Part model, mm, in its own coordinate system. Round coordinates to 2 decimals unless told otherwise and drop trailing zeros. Loops run counter-clockwise (first coordinate to the right, second up) from the corner with the lowest first, then second, coordinate; pieces in that order, holes last.
from build123d import *

# Parameters (mm, degrees)
SKETCH1_R           = 14.5
BOSS_EXTRUDE1_DEPTH = 50
SKETCH2_R           = 1.1
CUT_EXTRUDE1_DEPTH  = 47
CHAMFER1_SIZE       = 0.5


with BuildPart() as part:
    # Sketch1 → Boss-Extrude1 (new body)
    with BuildSketch(Plane(origin=(0, 0, 0), x_dir=(1, 0, 0), z_dir=(0, 1, 0))):
        with Locations(Location((0, 0, 0), (0, 0, 270))):
            Circle(SKETCH1_R)
    extrude(amount=BOSS_EXTRUDE1_DEPTH)

    # Sketch2 → Cut-Extrude1 (cut)
    with BuildSketch(Plane.XZ):
        with BuildLine():
            Line((-12.75, 0.9), (-12.75, -0.9))
            Line((-12.75, -0.9), (-11.638182396, -0.9))
            ThreePointArc((-11.638182396, -0.9), (-12.005537317, -1.66663011), (-12.573189655, -2.299435125))
            ThreePointArc((-12.573189655, -2.299435125), (-9.280361808, -8.789049136), (-2.979270067, -12.429660087))
            ThreePointArc((-2.979270067, -12.429660087), (0, -9.781725236), (2.979270067, -12.429660087))
            ThreePointArc((2.979270067, -12.429660087), (9.280361808, -8.789049136), (12.573189655, -2.299435125))
            ThreePointArc((12.573189655, -2.299435125), (12.005537317, -1.66663011), (11.638182396, -0.9))
            Line((11.638182396, -0.9), (12.75, -0.9))
            Line((12.75, -0.9), (12.75, 0.9))
            Line((12.75, 0.9), (11.638182396, 0.9))
            ThreePointArc((11.638182396, 0.9), (12.005537317, 1.66663011), (12.573189655, 2.299435125))
            ThreePointArc((12.573189655, 2.299435125), (9.280361808, 8.789049136), (2.979270067, 12.429660087))
            ThreePointArc((2.979270067, 12.429660087), (0, 9.781725236), (-2.979270067, 12.429660087))
            ThreePointArc((-2.979270067, 12.429660087), (-9.280361808, 8.789049136), (-12.573189655, 2.299435125))
            ThreePointArc((-12.573189655, 2.299435125), (-12.005537317, 1.66663011), (-11.638182396, 0.9))
            Line((-11.638182396, 0.9), (-12.75, 0.9))
        make_face()
        with Locations(Location((0, -12.781725236, 0), (0, 0, 270))):
            Circle(SKETCH2_R)
        with Locations(Location((0, 12.781725236, 0), (0, 0, 270))):
            Circle(SKETCH2_R)
    extrude(amount=-CUT_EXTRUDE1_DEPTH, mode=Mode.SUBTRACT)

    # Chamfer1
    chamfer1_edges = [part.edges().sort_by_distance(p)[0] for p in [
        (9.280361808, 47, 8.789049136),
        (0, 0, -14.5),
        (12.75, 47, 0),
        (-9.280361808, 47, -8.789049136),
        (-12.75, 47, 0),
        (-9.280361808, 0, -8.789049136),
        (9.280361808, 0, -8.789049136),
        (9.280361808, 0, 8.789049136),
        (-9.280361808, 0, 8.789049136),
        (0, 50, -14.5),
    ]]
    chamfer(chamfer1_edges, length=CHAMFER1_SIZE)


solid = part.part
1) Drop flat-ended pins along their axis: pin 1 Ø5 at (y, z) = (30.5, -4) entering from +X; pin 2 Ø4 at (y, z) = (28, 8.5) entering from -X; pin 3 Ø3 at (x, z) = (-4.5, 3) entering from -Y. Give the stop position or say it passes through.
Values:
pin 1: stops at x = 14.42
pin 2: stops at x = -12.96
pin 3: stops at y = 47
2) Slice it at B-B, the plane z = 0. Give the cut face in (x, y).
Values:
outline: (-14.5, 0.5) - (-14, 0) - (-12.75, 0) - (-12.75, 46.5) - (-12.25, 47) - (12.25, 47) - (12.75, 46.5) - (12.75, 0) - (14, 0) - (14.5, 0.5) - (14.5, 49.5) - (14, 50) - (-14, 50) - (-14.5, 49.5) - close
3) Slice it at C-C, the plane x = 0. Give the cut face in (y, z), then the cut area to 3 significant figures.
Values:
outline: (0, -14) - (0.5, -14.5) - (49.5, -14.5) - (50, -14) - (50, 14) - (49.5, 14.5) - (0.5, 14.5) - (0, 14) - (0, 13.88) - (47, 13.88) - (47, 11.68) - (0, 11.68) - (0, 9.78) - (47, 9.78) - (47, -9.78) - (0, -9.78) - (0, -11.68) - (47, -11.68) - (47, -13.88) - (0, -13.88) - close
area: 323 mm2
4) Slice it at A-A, the plane y = 19. Give the cut face in (x, z).
Values:
outline: circle Ø29 at (0, 0); hole (-12.75, -0.9) - (-11.64, -0.9) arc R3 cw to (-12.57, -2.3) arc R12.78 ccw to (-2.98, -12.43) arc R3 cw to (2.98, -12.43) arc R12.78 ccw to (12.57, -2.3) arc R3 cw to (11.64, -0.9) - (12.75, -0.9) - (12.75, 0.9) - (11.64, 0.9) arc R3 cw to (12.57, 2.3) arc R12.78 ccw to (2.98, 12.43) arc R3 cw to (-2.98, 12.43) arc R12.78 ccw to (-12.57, 2.3) arc R3 cw to (-11.64, 0.9) - (-12.75, 0.9) - close; hole circle Ø2.2 at (0, -12.78); hole circle Ø2.2 at (0, 12.78)
5) Wall check: line 1 along X through (y, z) = (35.5, 2.5); line 2 along X through (y, z) = (37.5, 4.75); line 3 along Z through (x, y) = (4, 18). Give the ranges that are in metal, low to high.
Values:
line 1: x = -14.28 to -12.53, 12.53 to 14.28
line 2: x = -13.7 to -11.87, 11.87 to 13.7
line 3: z = -13.94 to -12.14, 12.14 to 13.94
6) Mould opens along X. For faces 1 (the face through (-5.554, 24.657, 13.394)), 2 (the face through (0, 50, 0)), 3 (the face through (9.417, 0.365, 8.842)) say: released by +X, released by -X, zero draft, split by the parting line, or undercut.
Values:
face 1: split by the parting line
face 2: zero draft
face 3: undercut
